Geometry check sheet. Reference: the model listing, model coordinates, mm. A direction names the side the tool comes from. Give positions to 0.01 mm unless a question says otherwise; leave off trailing zeros. Order: outer loops, then holes, each group sorted by start corner. A loop starts at its lowest first (then second) coordinate and runs counter-clockwise, first axis right, second up.
from build123d import *

# Parameters (mm, degrees)
SKETCH2_R          = 2
CUT_EXTRUDE1_DEPTH = 6


with BuildPart() as part:
    # Sketch1 → Revolve1 (revolve)
    with BuildSketch(Plane.XY, mode=Mode.PRIVATE) as revolve1_sk:
        Polygon((0, 0), (0, 37), (2, 37), (2, 25.684518386), (3, 25.684518386), (3, 17.191909634), (8, 17.191909634), (8, 15.191909634), (3, 15.191909634), (3, 0), align=None)
    revolve(revolve1_sk.sketch.rotate(Axis((0, 0, 0), (0, 1, 0)), 90), axis=Axis((0, 0, 0), (0, 1, 0)))

    # Sketch2 → Cut-Extrude1 (cut)
    with BuildSketch(Plane.XZ):
        with Locations(Location((0, 0, 0), (0, 0, 270))):
            Circle(SKETCH2_R)
    extrude(amount=-CUT_EXTRUDE1_DEPTH, mode=Mode.SUBTRACT)


solid = part.part
Item 1: Sectioned sample at C-C (y = 5). Enter the section's corners in (x, z), and give its area (3 significant figures).
Reported:
outline: circle Ø6 at (0, 0); hole circle Ø4 at (0, 0)
area: 15.7 mm2
Item 2: Sectioned sample at A-A (x = 0). Enter the section's corners in (y, z).
Reported:
outline: (0, -3) - (15.19, -3) - (15.19, -8) - (17.19, -8) - (17.19, -3) - (25.68, -3) - (25.68, -2) - (37, -2) - (37, 2) - (25.68, 2) - (25.68, 3) - (17.19, 3) - (17.19, 8) - (15.19, 8) - (15.19, 3) - (0, 3) - (0, 2) - (6, 2) - (6, -2) - (0, -2) - close
Item 3: Set-up check for faces 5 (the flat face through (2, 25.685, 1)), 6 (the flat face through (-0.1, 15.192, -3.4)), 7 (the cylindrical face through (7.81, 16.18, 1.73)): record each of +Z, -Z, +X, -X, +Y, -Y from which the full face is reachable in a straight line by a thin tool's end or side.
Reported:
face 5: +Y
face 6: -Y
face 7: +Y, -Y
Item 4: Sectioned sample at D-D (y = 21). Enter the section's corners in (x, z).
Reported:
outline: circle Ø6 at (0, 0)
Item 5: Scan lines: L1, parallel to X at y = 2.7, z = 0; L2, parallel to Y at x = 1, z = -2.5; L3, parallel to Y at x = 4.5, z = -3.25. Record each from-to range of solid material in increasing order.
Reported:
L1: x = -3 to -2, 2 to 3
L2: y = 0 to 25.68
L3: y = 15.19 to 17.19
Item 6: Gauge pin test, flat ends, axial feed: pin 1 (3 mm diameter, centred on x = -0.5, y = 10.5, fed in from +Z); pin 2 (5 mm diameter, centred on y = 5.5, z = -4, fed in from -X); pin 3 (2 mm diameter, centred on x = -0.5, z = 0, fed in from -Y). Record the tip position at first contact, or that the pin passes through.
Reported:
pin 1: stops at z = 3
pin 2: stops at x = -2.6
pin 3: stops at y = 6
Item 7: Sectioned sample at B-B (z = 0). Enter the section's corners in (x, y).
Reported:
outline: (-8, 15.19) - (-3, 15.19) - (-3, 0) - (-2, 0) - (-2, 6) - (2, 6) - (2, 0) - (3, 0) - (3, 15.19) - (8, 15.19) - (8, 17.19) - (3, 17.19) - (3, 25.68) - (2, 25.68) - (2, 37) - (-2, 37) - (-2, 25.68) - (-3, 25.68) - (-3, 17.19) - (-8, 17.19) - close
Item 8: Draft check along X on faces 1 (the flat face through (0, 6, 0)), 2 (the cylindrical face through (2, 31, 0)), 3 (the cylindrical face through (-2, 3, 0)), 4 (the flat face through (-0.1, 17.192, 3.4)). Enter one of: released by +X, released by -X, zero draft, split by the parting line, or undercut.
Reported:
face 1: undercut
face 2: split by the parting line
face 3: undercut
face 4: zero draft
